from build123d import *

# Parameters (mm, degrees)
SKETCH1_W            = 111.1
SKETCH1_H            = 60
BOSS_EXTRUDE1_DEPTH  = 3
SKETCH2_W            = 111.1
SKETCH2_H            = 60
SKETCH2_W_2          = 105.3
SKETCH2_H_2          = 55
BOSS_EXTRUDE2_DEPTH  = 40.5
SKETCH5_R            = 21
BOSS_EXTRUDE4_DEPTH  = 15
SKETCH6_W            = 15.5
SKETCH6_H            = 37
CUT_EXTRUDE1_DEPTH   = 21
BOSS_EXTRUDE5_START  = -1
SKETCH8_R            = 21
SKETCH8_W            = 12.3
SKETCH8_H            = 34.3
BOSS_EXTRUDE5_DEPTH  = 1
BOSS_EXTRUDE6_START  = -1
SKETCH9_R            = 21
SKETCH9_W            = 12.3
SKETCH9_H            = 34.3
BOSS_EXTRUDE6_DEPTH  = 1
SKETCH10_W           = 126.244554882
SKETCH10_H           = 68.697179438
CUT_EXTRUDE3_DEPTH   = 53
SKETCH12_W           = 1
SKETCH12_H           = 1.5
BOSS_EXTRUDE8_DEPTH  = 2
FILLET1_R            = 2
SKETCH13_R           = 6
SKETCH13_R_2         = 2.5
CUT_EXTRUDE4_DEPTH   = 14
SKETCH15_W           = 3
SKETCH15_H           = 10
BOSS_EXTRUDE9_DEPTH  = 40.5
SKETCH16_R           = 3.5
CUT_EXTRUDE5_DEPTH   = 1
SKETCH17_W           = 7
SKETCH17_H           = 11
BOSS_EXTRUDE10_DEPTH = 14
SKETCH18_W           = 7
SKETCH18_H           = 1.5
CUT_EXTRUDE6_DEPTH   = 14
SKETCH19_R           = 3.5
SKETCH19_R_2         = 2.5
BOSS_EXTRUDE11_DEPTH = 5


with BuildPart() as part:
    # Sketch1 → Boss-Extrude1 (new body)
    with BuildSketch(Plane(origin=(0, 0, 0), x_dir=(1, 0, 0), z_dir=(0, 1, 0))):
        Rectangle(SKETCH1_W, SKETCH1_H)
    extrude(amount=BOSS_EXTRUDE1_DEPTH)

    # Sketch2 → Boss-Extrude2 (add)
    with BuildSketch(Plane(origin=(0, 3, 0), x_dir=(1, 0, 0), z_dir=(0, 1, 0))):
        Rectangle(SKETCH2_W, SKETCH2_H)
        Rectangle(SKETCH2_W_2, SKETCH2_H_2, mode=Mode.SUBTRACT)
    extrude(amount=BOSS_EXTRUDE2_DEPTH)

    # Sketch5 → Boss-Extrude4 (add)
    with BuildSketch(Plane(origin=(0, 0, -30), x_dir=(-1, 0, 0), z_dir=(0, 0, -1))):
        with Locations((-27.775, 21.75)):
            Circle(SKETCH5_R)
        with Locations(Location((27.775, 21.75, 0), (0, 0, 180))):
            Circle(SKETCH5_R)
    extrude(amount=BOSS_EXTRUDE4_DEPTH)

    # Sketch6 → Cut-Extrude1 (cut)
    with BuildSketch(Plane(origin=(0, 0, -45), x_dir=(-1, 0, 0), z_dir=(0, 0, -1))):
        with Locations((-27.775, 21.75)):
            Rectangle(SKETCH6_W, SKETCH6_H)
        with Locations((27.775, 21.75)):
            Rectangle(SKETCH6_W, SKETCH6_H)
    extrude(amount=-CUT_EXTRUDE1_DEPTH, mode=Mode.SUBTRACT)

    # Sketch8 → Boss-Extrude5 (add)
    with BuildSketch(Plane(origin=(0, 0, -45), x_dir=(-1, 0, 0), z_dir=(0, 0, -1)).offset(BOSS_EXTRUDE5_START)):
        with Locations((-27.775, 21.75)):
            Circle(SKETCH8_R)
        with Locations((-27.775, 21.75)):
            Rectangle(SKETCH8_W, SKETCH8_H, mode=Mode.SUBTRACT)
    extrude(amount=BOSS_EXTRUDE5_DEPTH)

    # Sketch9 → Boss-Extrude6 (add)
    with BuildSketch(Plane(origin=(0, 0, -45), x_dir=(-1, 0, 0), z_dir=(0, 0, -1)).offset(BOSS_EXTRUDE6_START)):
        with Locations(Location((27.775, 21.75, 0), (0, 0, 180))):
            Circle(SKETCH9_R)
        with Locations((27.775, 21.75)):
            Rectangle(SKETCH9_W, SKETCH9_H, mode=Mode.SUBTRACT)
    extrude(amount=BOSS_EXTRUDE6_DEPTH)

    # Sketch10 → Cut-Extrude3 (cut)
    with BuildSketch(Plane.XY.offset(-27.5)):
        with Locations((0, 21.75)):
            Rectangle(SKETCH10_W, SKETCH10_H)
    extrude(amount=-CUT_EXTRUDE3_DEPTH, mode=Mode.SUBTRACT)

    # Sketch12 → Boss-Extrude8 (add)
    with BuildSketch(Plane(origin=(0, 0, -27.5), x_dir=(-1, 0, 0), z_dir=(0, 0, -1))):
        with Locations((52.15, 18.9)):
            Rectangle(SKETCH12_W, SKETCH12_H)
        with Locations((52.15, 7.95)):
            Rectangle(SKETCH12_W, SKETCH12_H)
        with Locations((-52.15, 18.9)):
            Rectangle(SKETCH12_W, SKETCH12_H)
        with Locations((-52.15, 24.6)):
            Rectangle(SKETCH12_W, SKETCH12_H)
        with Locations((52.15, 24.6)):
            Rectangle(SKETCH12_W, SKETCH12_H)
        with Locations((-52.15, 7.95)):
            Rectangle(SKETCH12_W, SKETCH12_H)
    extrude(amount=-BOSS_EXTRUDE8_DEPTH)

    # Fillet1
    fillet1_edges = [part.edges().sort_by_distance(p)[0] for p in [
        (55.55, 21.75, 30),
        (-55.55, 21.75, 30),
    ]]
    fillet(fillet1_edges, radius=FILLET1_R)

    # Sketch13 → Cut-Extrude4 (cut)
    with BuildSketch(Plane(origin=(-52.65, 0, 0), x_dir=(0, 0, -1), z_dir=(1, 0, 0))):
        with Locations((12.5, 32.625)):
            Circle(SKETCH13_R)
        with Locations((12.5, 10.875)):
            Circle(SKETCH13_R)
        with Locations((5, 21.75)):
            Circle(SKETCH13_R_2)
        with BuildLine():
            Line((-25, 25.75), (-27, 25.75))
            ThreePointArc((-27, 25.75), (-27.707106781, 25.457106781), (-28, 24.75))
            Line((-28, 24.75), (-28, 18.75))
            ThreePointArc((-28, 18.75), (-27.707106781, 18.042893219), (-27, 17.75))
            Line((-27, 17.75), (-25, 17.75))
            ThreePointArc((-25, 17.75), (-24.292893219, 18.042893219), (-24, 18.75))
            Line((-24, 18.75), (-24, 24.75))
            ThreePointArc((-24, 24.75), (-24.292893219, 25.457106781), (-25, 25.75))
        make_face()
    extrude(amount=-CUT_EXTRUDE4_DEPTH, mode=Mode.SUBTRACT)

    # Sketch15 → Boss-Extrude9 (add)
    with BuildSketch(Plane(origin=(0, 3, 0), x_dir=(1, 0, 0), z_dir=(0, 1, 0))):
        with Locations((-41.85, 12.5)):
            Rectangle(SKETCH15_W, SKETCH15_H)
    extrude(amount=BOSS_EXTRUDE9_DEPTH)

    # Sketch16 → Cut-Extrude5 (cut)
    with BuildSketch(Plane.ZY.offset(55.55)):
        with Locations((-5, 21.75)):
            Circle(SKETCH16_R)
    extrude(amount=-CUT_EXTRUDE5_DEPTH, mode=Mode.SUBTRACT)

    # Sketch17 → Boss-Extrude10 (add)
    with BuildSketch(Plane(origin=(0, 0, 27.5), x_dir=(-1, 0, 0), z_dir=(0, 0, -1))):
        with Locations((-49.15, 23.25)):
            Rectangle(SKETCH17_W, SKETCH17_H)
    extrude(amount=BOSS_EXTRUDE10_DEPTH)

    # Sketch18 → Cut-Extrude6 (cut)
    with BuildSketch(Plane(origin=(0, 0, 27.5), x_dir=(-1, 0, 0), z_dir=(0, 0, -1))):
        with Locations((-49.15, 29.5)):
            Rectangle(SKETCH18_W, SKETCH18_H)
        with Locations((-49.15, 17)):
            Rectangle(SKETCH18_W, SKETCH18_H)
    extrude(amount=-CUT_EXTRUDE6_DEPTH, mode=Mode.SUBTRACT)

    # Sketch19 → Boss-Extrude11 (add)
    with BuildSketch(Plane(origin=(-52.65, 0, 0), x_dir=(0, 0, -1), z_dir=(1, 0, 0))):
        with Locations(Location((5, 21.75, 0), (0, 0, 180))):
            Circle(SKETCH19_R)
        with Locations((5, 21.75)):
            Circle(SKETCH19_R_2, mode=Mode.SUBTRACT)
    extrude(amount=BOSS_EXTRUDE11_DEPTH)


solid = part.part
Verification items for the finished model (mm, model axes). A direction names the side the tool comes from. Give positions to 0.01 mm unless a question says otherwise; leave off trailing zeros. Loops run counter-clockwise (first coordinate to the right, second up) from the corner with the lowest first, then second, coordinate; pieces in that order, holes last. Notation, with made-up numbers: (80, -10) - (135, -10) arc R27 ccw to (135, 21) - close; hole circle Ø2 at (-15.75, 73.25). An arc over 180 degrees is marked (long way). Write each question's results on one line, items separated by ' | '.
1) Material ranges on L1, parallel to Y at x = -54, z = -12; L2, parallel to Y at x = -51.2, z = -5; L3, parallel to X at y = 22, z = -18.5, recorded low to high. Write a range as from..to.
Solution:
L1: 0..4.9, 16.85..26.65, 38.6..43.5 | L2: 0..3, 18.25..19.25, 24.25..25.25 | L3: -55.55..-52.65, 52.65..55.55
2) Sectioned sample at B-B on z = -12.5. Record the boundary of the cut face in (x, y) (3 decimals), plus the area to 3 significant figures.
Solution:
outline: (-55.55, 0) - (55.55, 0) - (55.55, 43.5) - (52.65, 43.5) - (52.65, 3) - (-40.35, 3) - (-40.35, 43.5) - (-43.35, 43.5) - (-43.35, 3) - (-52.65, 3) - (-52.65, 4.875) - (-55.55, 4.875) - close; (-55.55, 16.875) - (-52.65, 16.875) - (-52.65, 26.625) - (-55.55, 26.625) - close; (-55.55, 38.625) - (-52.65, 38.625) - (-52.65, 43.5) - (-55.55, 43.5) - close | area: 620 mm2
3) Depth check by flat-ended pin: P1, Ø7.5, axis at x = 48.5, z = 23, coming from the +Y side; P2, Ø1.5, axis at x = -20.5, y = 27.5, coming from the -Z side; P3, Ø6, axis at y = 21.75, z = -5, coming from the -X side. Enter the tip coordinate at first touch or a pass-through.
Solution:
P1: y = 28.75 | P2: z = 27.5 | P3: x = -54.55
4) Tool access check on faces 1 (the flat face through (-54, 25.75, 26)), 2 (the flat face through (49, 16.25, 29)), 3 (the cylindrical face through (-50.18, 18.28, -5.46)), 4 (the flat face through (-43.35, 23, -12)). Record the directions out of +Z, -Z, +X, -X, +Y, -Y that give a thin tool (end or side, any length) a straight path to the whole face; none if there is none.
Solution:
face 1: -X | face 2: +Z, -Z | face 3: none | face 4: -Z, +Y
5) Sectioned sample at D-D on y = 34.5. Record the boundary of the cut face in (x, z).
Solution:
outline: (-55.55, -27.5) - (-52.65, -27.5) - (-52.65, -18.2) - (-55.55, -18.2) - close; (-55.55, -6.8) - (-52.65, -6.8) - (-52.65, 27.5) - (52.65, 27.5) - (52.65, -27.5) - (55.55, -27.5) - (55.55, 28) arc R2 ccw to (53.55, 30) - (-53.55, 30) arc R2 ccw to (-55.55, 28) - close; (-43.35, -17.5) - (-40.35, -17.5) - (-40.35, -7.5) - (-43.35, -7.5) - close
6) Mould release check, pull along Y, two halves, no side actions. Record for faces 5 (the flat face through (-42, 23, -7.5)), 6 (the flat face through (-54.55, 19.5, -3.5)), 7 (the flat face through (0, 43.5, 29)): pulls with the +Y half, pulls with the -Y half, needs draft (parallel to the pull), parting line crosses it, or undercut.
Solution:
face 5: needs draft | face 6: undercut | face 7: pulls with the +Y half
7) Sectioned sample at C-C on z = -5. Record the boundary of the cut face in (x, y).
Solution:
outline: (-55.55, 0) - (55.55, 0) - (55.55, 43.5) - (52.65, 43.5) - (52.65, 3) - (-52.65, 3) - (-52.65, 18.25) - (-47.65, 18.25) - (-47.65, 19.25) - (-54.55, 19.25) - (-54.55, 18.25) - (-55.55, 18.25) - close; (-55.55, 25.25) - (-54.55, 25.25) - (-54.55, 24.25) - (-47.65, 24.25) - (-47.65, 25.25) - (-52.65, 25.25) - (-52.65, 43.5) - (-55.55, 43.5) - close
8) Sectioned sample at A-A on y = 21.75. Count the separate pieces of the cut face and the enclosed holes in it, plus the area to 3 significant figures.
Solution:
separate pieces: 4 | enclosed holes: 0 | area: 705 mm2
